from build123d import *

# Parameters (mm, degrees)
ESQUISSE1_R             = 2.5
BASE_EXTRUSION_DEPTH    = 2.5
ESQUISSE2_R             = 1.5
BOSS_EXTRU_1_DEPTH      = 10
ENL_V_MAT_EXTRU_1_DEPTH = 2
CONG_1_R                = 0.5
CHANFREIN1_SIZE         = 0.5


with BuildPart() as part:
    # Esquisse1 → Base-Extrusion (new body)
    with BuildSketch(Plane.XY):
        Circle(ESQUISSE1_R)
    extrude(amount=BASE_EXTRUSION_DEPTH)

    # Esquisse2 → Boss.-Extru.1 (add)
    with BuildSketch(Plane.XY.offset(2.5)):
        Circle(ESQUISSE2_R)
    extrude(amount=BOSS_EXTRU_1_DEPTH)

    # Esquisse3 → Enlèv. mat.-Extru.1 (cut)
    with BuildSketch(Plane(origin=(0, 0, 0), x_dir=(-1, 0, 0), z_dir=(0, 0, -1))):
        Polygon((0, 1.45), (-1.25, 0.728312164), (-1.25, -0.715063509), (0, -1.436751346), (1.25, -0.715063509), (1.25, 0.728312164), align=None)
    extrude(amount=-ENL_V_MAT_EXTRU_1_DEPTH, mode=Mode.SUBTRACT)

    # Congé1
    cong_1_edges = [part.edges().sort_by_distance(p)[0] for p in [
        (-2.5, 0, 0),
    ]]
    fillet(cong_1_edges, radius=CONG_1_R)

    # Chanfrein1
    chanfrein1_edges = [part.edges().sort_by_distance(p)[0] for p in [
        (-1.5, 0, 12.5),
    ]]
    chamfer(chanfrein1_edges, length=CHANFREIN1_SIZE)


solid = part.part
The model under review builds one solid part; all positions refer to its coordinate system, in mm. A direction names the side the tool comes from. Round coordinates to 2 decimals unless told otherwise and drop trailing zeros. Order: outer loops, then holes, each group sorted by start corner. A loop starts at its lowest first (then second) coordinate and runs counter-clockwise, first axis right, second up. Notation, with made-up numbers: (6.5, -3) -> (45.5, -3) arc R5 ccw to (45.5, 3) -> close; hole circle Ø11 at (6.25, -32.5). An arc over 180 degrees is marked (long way). Write item = value, one per line. Start each with the question number.
Item 1: Consider section A-A on y = 0. Write out the cut boundary in (x, z).
Item 2: For line 1 along X through (y, z) = (-2, 2); line 2 along X through (y, z) = (-0.9, 11); line 3 along Y through (x, z) = (1.15, 7.75), list the stretches that pass through material, from the lowest coordinate up.
Item 3: Mouldability with a two-part tool opening along Y and no side actions: class faces 3 (the face through (-1.5, 0.07, 7.18)), 4 (the face through (0, -2, 2.5)), 5 (the face through (0.62, 1.09, 0.99)) as released by +Y, released by -Y, zero draft, split by the parting line, or undercut.
Item 4: Consider section B-B on z = 7.5. Write out the cut boundary in (x, y), plus the area to 3 significant figures.
Item 5: For faces 1 (the face through (-0.54, -2.44, 1.49)), 2 (the face through (1.25, 0, 1)), list the 3-axis set-ups (+Z, -Z, +X, -X, +Y, -Y) from which the entire face can be reached by the end or side of a thin tool; tool diameter is ignored.
Item 6: Clearance check with flat-ended pins moving along their axes: pin 1 Ø0.7 at (y, z) = (0.5, 1) entering from -X; pin 2 Ø2 at (x, z) = (2, 7) entering from +Y; pin 3 Ø3 at (x, y) = (1, -1.5) entering from -Z; pin 4 Ø1.5 at (y, z) = (-1, 8.5) entering from -X. State where each tip first meets the part, or that it passes through.
Conclusion:
q1.outline = (-2.5, 0.5) arc R0.5 ccw to (-2, 0) -> (-1.25, 0) -> (-1.25, 2) -> (1.25, 2) -> (1.25, 0) -> (2, 0) arc R0.5 ccw to (2.5, 0.5) -> (2.5, 2.5) -> (1.5, 2.5) -> (1.5, 12) -> (1, 12.5) -> (-1, 12.5) -> (-1.5, 12) -> (-1.5, 2.5) -> (-2.5, 2.5) -> close
q2.line_1 = -1.5 to 1.5
q2.line_2 = -1.2 to 1.2
q2.line_3 = -0.96 to 0.96
q3.face_3 = split by the parting line
q3.face_4 = zero draft
q3.face_5 = undercut
q4.outline = circle Ø3 at (0, 0)
q4.area = 7.07 mm2
q5.face_1 = +Z, -Z
q5.face_2 = -Z
q6.pin_1 = -2.5
q6.pin_2 = 1.12
q6.pin_3 = 0
q6.pin_4 = -1.48
